Can you work these out from the model? Positions are in its coordinate system, mm. A direction names the side the tool comes from. Give positions to 0.01 mm unless a question says otherwise; leave off trailing zeros. Loops run counter-clockwise (first coordinate to the right, second up) from the corner with the lowest first, then second, coordinate; pieces in that order, holes last. Notation, with made-up numbers: (83, 1.25) - (88, 1.25) arc R7 cw to (88, 5.25) - close; hole circle Ø7 at (-30.75, 81). An arc over 180 degrees is marked (long way). Write item = value, one per line.
from build123d import *

# Parameters (mm, degrees)
MODEL_R             = 57.954171366
MODEL_R_2           = 2.55
MODEL_R_3           = 5.5
BOSS_EXTRUDE1_DEPTH = 6.6


with BuildPart() as part:
    # Model → Boss-Extrude1 (new body)
    with BuildSketch(Plane.XY):
        with BuildLine():
            Line((93.9, 110.423468713), (91.4, 113.2))
            Line((91.4, 113.2), (-91.123468713, 113.2))
            Line((-91.123468713, 113.2), (-93.9, 110.7))
            Line((-93.9, 110.7), (-93.9, 100.5))
            Line((-93.9, 100.5), (-97.9, 100.5))
            ThreePointArc((-97.9, 100.5), (-99.667766953, 99.767766953), (-100.4, 98))
            Line((-100.4, 98), (-100.4, 83))
            ThreePointArc((-100.4, 83), (-99.667766953, 81.232233047), (-97.9, 80.5))
            Line((-97.9, 80.5), (-93.9, 80.5))
            Line((-93.9, 80.5), (-93.9, 75.1))
            Line((-93.9, 75.1), (-82.9, 75.1))
            Line((-82.9, 75.1), (-82.9, 76.685))
            ThreePointArc((-82.9, 76.685), (-82.753553391, 77.038553391), (-82.4, 77.185))
            Line((-82.4, 77.185), (-78.4, 77.185))
            ThreePointArc((-78.4, 77.185), (-78.046446609, 77.038553391), (-77.9, 76.685))
            Line((-77.9, 76.685), (-77.9, 75.1))
            Line((-77.9, 75.1), (-73.4, 75.1))
            ThreePointArc((-73.4, 75.1), (-73.046446609, 74.953553391), (-72.9, 74.6))
            Line((-72.9, 74.6), (-72.9, 72.05))
            ThreePointArc((-72.9, 72.05), (-73.046446609, 71.696446609), (-73.4, 71.55))
            Line((-73.4, 71.55), (-77.9, 71.55))
            Line((-77.9, 71.55), (-77.9, 69.965))
            ThreePointArc((-77.9, 69.965), (-78.046446609, 69.611446609), (-78.4, 69.465))
            Line((-78.4, 69.465), (-82.4, 69.465))
            ThreePointArc((-82.4, 69.465), (-82.753553391, 69.611446609), (-82.9, 69.965))
            Line((-82.9, 69.965), (-82.9, 71.55))
            Line((-82.9, 71.55), (-93.9, 71.55))
            Line((-93.9, 71.55), (-93.9, -69.65))
            Line((-93.9, -69.65), (-82.9, -69.65))
            Line((-82.9, -69.65), (-82.9, -68.065))
            ThreePointArc((-82.9, -68.065), (-82.753553391, -67.711446609), (-82.4, -67.565))
            Line((-82.4, -67.565), (-78.4, -67.565))
            ThreePointArc((-78.4, -67.565), (-78.046446609, -67.711446609), (-77.9, -68.065))
            Line((-77.9, -68.065), (-77.9, -69.65))
            Line((-77.9, -69.65), (-73.4, -69.65))
            ThreePointArc((-73.4, -69.65), (-73.046446609, -69.796446609), (-72.9, -70.15))
            Line((-72.9, -70.15), (-72.9, -72.7))
            ThreePointArc((-72.9, -72.7), (-73.046446609, -73.053553391), (-73.4, -73.2))
            Line((-73.4, -73.2), (-77.9, -73.2))
            Line((-77.9, -73.2), (-77.9, -74.785))
            ThreePointArc((-77.9, -74.785), (-78.046446609, -75.138553391), (-78.4, -75.285))
            Line((-78.4, -75.285), (-82.4, -75.285))
            ThreePointArc((-82.4, -75.285), (-82.753553391, -75.138553391), (-82.9, -74.785))
            Line((-82.9, -74.785), (-82.9, -73.2))
            Line((-82.9, -73.2), (-93.9, -73.2))
            Line((-93.9, -73.2), (-93.9, -80.5))
            Line((-93.9, -80.5), (-97.9, -80.5))
            ThreePointArc((-97.9, -80.5), (-99.667766953, -81.232233047), (-100.4, -83))
            Line((-100.4, -83), (-100.4, -98))
            ThreePointArc((-100.4, -98), (-99.667766953, -99.767766953), (-97.9, -100.5))
            Line((-97.9, -100.5), (-93.9, -100.5))
            Line((-93.9, -100.5), (-93.9, -110.423468713))
            Line((-93.9, -110.423468713), (-91.4, -113.2))
            Line((-91.4, -113.2), (91.123468713, -113.2))
            Line((91.123468713, -113.2), (93.9, -110.7))
            Line((93.9, -110.7), (93.9, -100.5))
            Line((93.9, -100.5), (97.9, -100.5))
            ThreePointArc((97.9, -100.5), (99.667766953, -99.767766953), (100.4, -98))
            Line((100.4, -98), (100.4, -83))
            ThreePointArc((100.4, -83), (99.667766953, -81.232233047), (97.9, -80.5))
            Line((97.9, -80.5), (93.9, -80.5))
            Line((93.9, -80.5), (93.9, -73.2))
            Line((93.9, -73.2), (82.9, -73.2))
            Line((82.9, -73.2), (82.9, -74.785))
            ThreePointArc((82.9, -74.785), (82.753553391, -75.138553391), (82.4, -75.285))
            Line((82.4, -75.285), (78.4, -75.285))
            ThreePointArc((78.4, -75.285), (78.046446609, -75.138553391), (77.9, -74.785))
            Line((77.9, -74.785), (77.9, -73.2))
            Line((77.9, -73.2), (73.4, -73.2))
            ThreePointArc((73.4, -73.2), (73.046446609, -73.053553391), (72.9, -72.7))
            Line((72.9, -72.7), (72.9, -70.15))
            ThreePointArc((72.9, -70.15), (73.046446609, -69.796446609), (73.4, -69.65))
            Line((73.4, -69.65), (77.9, -69.65))
            Line((77.9, -69.65), (77.9, -68.065))
            ThreePointArc((77.9, -68.065), (78.046446609, -67.711446609), (78.4, -67.565))
            Line((78.4, -67.565), (82.4, -67.565))
            ThreePointArc((82.4, -67.565), (82.753553391, -67.711446609), (82.9, -68.065))
            Line((82.9, -68.065), (82.9, -69.65))
            Line((82.9, -69.65), (93.9, -69.65))
            Line((93.9, -69.65), (93.9, 71.55))
            Line((93.9, 71.55), (82.9, 71.55))
            Line((82.9, 71.55), (82.9, 69.965))
            ThreePointArc((82.9, 69.965), (82.753553391, 69.611446609), (82.4, 69.465))
            Line((82.4, 69.465), (78.4, 69.465))
            ThreePointArc((78.4, 69.465), (78.046446609, 69.611446609), (77.9, 69.965))
            Line((77.9, 69.965), (77.9, 71.55))
            Line((77.9, 71.55), (73.4, 71.55))
            ThreePointArc((73.4, 71.55), (73.046446609, 71.696446609), (72.9, 72.05))
            Line((72.9, 72.05), (72.9, 74.6))
            ThreePointArc((72.9, 74.6), (73.046446609, 74.953553391), (73.4, 75.1))
            Line((73.4, 75.1), (77.9, 75.1))
            Line((77.9, 75.1), (77.9, 76.685))
            ThreePointArc((77.9, 76.685), (78.046446609, 77.038553391), (78.4, 77.185))
            Line((78.4, 77.185), (82.4, 77.185))
            ThreePointArc((82.4, 77.185), (82.753553391, 77.038553391), (82.9, 76.685))
            Line((82.9, 76.685), (82.9, 75.1))
            Line((82.9, 75.1), (93.9, 75.1))
            Line((93.9, 75.1), (93.9, 80.5))
            Line((93.9, 80.5), (97.9, 80.5))
            ThreePointArc((97.9, 80.5), (99.667766953, 81.232233047), (100.4, 83))
            Line((100.4, 83), (100.4, 98))
            ThreePointArc((100.4, 98), (99.667766953, 99.767766953), (97.9, 100.5))
            Line((97.9, 100.5), (93.9, 100.5))
            Line((93.9, 100.5), (93.9, 110.423468713))
        make_face()
        with Locations((-10.493238984, -43.592)):
            Circle(MODEL_R, mode=Mode.SUBTRACT)
        with Locations((81.2, -90.5)):
            Circle(MODEL_R_2, mode=Mode.SUBTRACT)
        with Locations((81.2, 90.5)):
            Circle(MODEL_R_2, mode=Mode.SUBTRACT)
        with Locations((-81.2, 90.5)):
            Circle(MODEL_R_2, mode=Mode.SUBTRACT)
        with Locations((-81.2, -90.5)):
            Circle(MODEL_R_2, mode=Mode.SUBTRACT)
        with Locations((45.952001664, -10.724806781)):
            Circle(MODEL_R_3, mode=Mode.SUBTRACT)
    extrude(amount=BOSS_EXTRUDE1_DEPTH)


solid = part.part
Q1. Imagine slicing it at B-B, the plane x = -37.5. Write out the boundary of the cut face in (y, z).
Output:
outline = (-113.2, 0) - (-94.87, 0) - (-94.87, 6.6) - (-113.2, 6.6) - close; (7.68, 0) - (113.2, 0) - (113.2, 6.6) - (7.68, 6.6) - close
Q2. For pin 1 (1.3 mm diameter, centred on y = 70.5, z = 4, fed in from +X); pin 2 (1.2 mm diameter, centred on x = 97, z = 4.5, fed in from +Y); pin 3 (2 mm diameter, centred on x = -96.5, z = 4, fed in from -Y); pin 4 (2 mm diameter, centred on x = -7, y = 87.5, fed in from -Z), each with a flat end and sliding along its axis, tell me the tip position at first contact or that it passes through.
Output:
pin_1 = 93.9
pin_2 = 100.5
pin_3 = -100.5
pin_4 = 0
Q3. I need wall thicknesses on L1, parallel to Y at x = -90, z = 0.5; L2, parallel to Y at x = -81.2, z = 3 (3 decimals); L3, parallel to X at y = 90, z = 5. Which ranges of each line are inside material? Lowest first, please.
Output:
L1 = -113.2 to -73.2, -69.65 to 71.55, 75.1 to 113.2
L2 = -113.2 to -93.05, -87.95 to -75.285, -67.565 to 69.465, 77.185 to 87.95, 93.05 to 113.2
L3 = -100.4 to -83.7, -78.7 to 78.7, 83.7 to 100.4
Q4. Imagine slicing it at A-A, the plane y = 90.5. Write out the boundary of the cut face in (x, z).
Output:
outline = (-100.4, 0) - (-83.75, 0) - (-83.75, 6.6) - (-100.4, 6.6) - close; (-78.65, 0) - (78.65, 0) - (78.65, 6.6) - (-78.65, 6.6) - close; (83.75, 0) - (100.4, 0) - (100.4, 6.6) - (83.75, 6.6) - close
Q5. Imagine slicing it at D-D, the plane y = 31.5. Write out the boundary of the cut face in (x, z).
Output:
outline = (-93.9, 0) - (93.9, 0) - (93.9, 6.6) - (-93.9, 6.6) - close
Q6. We'd pull the mould along Y, two halves only. Please class faces 5 (the flat face through (-100.4, -90, 3)), 6 (the flat face through (-88, 75.1, 3)), 7 (the flat face through (1, 113.2, 3)): released by +Y, released by -Y, zero draft, split by the parting line, or undercut.
Output:
face_5 = zero draft
face_6 = undercut
face_7 = released by +Y
Q7. Imagine slicing it at C-C, the plane y = -33.5. Write out the boundary of the cut face in (x, z).
Output:
outline = (-93.9, 0) - (-67.56, 0) - (-67.56, 6.6) - (-93.9, 6.6) - close; (46.58, 0) - (93.9, 0) - (93.9, 6.6) - (46.58, 6.6) - close
Q8. Which directions (+Z, -Z, +X, -X, +Y, -Y) give clear straight access to the entire face, cutting with the end or side of a thin tool? Please do faces 1 (the flat face through (-93.9, -105, 3)), 2 (the flat face through (88, 71.55, 3)), 3 (the flat face through (-93.9, 106, 3)), 4 (the flat face through (-93.9, 2, 3)).
Output:
face_1 = +Z, -Z, -X, -Y
face_2 = +Z, -Z, +X
face_3 = +Z, -Z, -X, +Y
face_4 = +Z, -Z, -X
